The model under review builds one solid part; all positions refer to its coordinate system, in mm. Face numbers are marked on the shaded views. A direction names the side the tool comes from. Coordinates: 2 decimals unless noted, no trailing zeros. Loops run counter-clockwise (first coordinate to the right, second up) from the corner with the lowest first, then second, coordinate; pieces in that order, holes last. Notation, with made-up numbers: (-20, 54) - (8, 54) arc R27 cw to (8, 76) - close; hole circle Ø2 at (42.5, 68). An arc over 180 degrees is marked (long way). Use a Markdown table: item, result. Add a question column.
1) To check wall thickness, follow L1, parallel to X at y = 4, z = 14; L2, parallel to Z at x = 12, y = 7.5; L3, parallel to X at y = 80, z = 5.5. State the ranges of each line that lie inside material, in increasing order. Write a range as [from, to].
2) Add section A-A, the plane z = 14. Give the boundary of the cut face in (x, y), and give its area (3 significant figures).
3) Add section C-C, the plane x = 2.75. Give the boundary of the cut face in (y, z).
4) For the marked faces 1, 2 and 3, list the 3-axis set-ups (+Z, -Z, +X, -X, +Y, -Y) from which the entire face can be reached by the end or side of a thin tool; tool diameter is ignored.
5) Add section B-B, the plane x = 12. Give the boundary of the cut face in (y, z), and give its area (3 significant figures).
6) Clearance check with flat-ended pins moving along their axes: pin 1 (6 mm diameter, centred on y = 53.5, z = 7, fed in from +X); pin 2 (10 mm diameter, centred on y = 52.5, z = -0.5, fed in from -X); pin 3 (4 mm diameter, centred on x = 3.5, y = 72.5, fed in from +Z). State where each tip first meets the part, or that it passes through.
7) Add section D-D, the plane y = 41. Give the boundary of the cut face in (x, z), and give its area (3 significant figures).
```python
from build123d import *

# Parameters (mm, degrees)
BOSS_EXTRUDE2_DEPTH = 150
SKETCH3_W           = 29.65685425
SKETCH3_H           = 33.65685425
SKETCH3_R           = 2
BOSS_EXTRUDE3_DEPTH = 10


with BuildPart() as part:
    # Sketch1 → Boss-Extrude2 (new body)
    with BuildSketch(Plane(origin=(0, 0, 0), x_dir=(1, 0, 0), z_dir=(0, 1, 0))):
        Polygon((-10, 12.5), (-10, -12.5), (10, -12.5), (10, -5), (8, -5), (8, -8.6), (0, -8.6), (-6.2, -6), (-6.2, 0), (-6.2, 6), (0, 8.6), (8, 8.6), (8, 5), (10, 5), (10, 12.5), align=None)
    extrude(amount=BOSS_EXTRUDE2_DEPTH)

    # Sketch3 → Boss-Extrude3 (add)
    with BuildSketch(Plane(origin=(0, 0, 0), x_dir=(1, 0, 0), z_dir=(0, 1, 0))):
        Rectangle(SKETCH3_W, SKETCH3_H)
        with Locations(Location((-12, 14, 0), (0, 0, 270))):
            Circle(SKETCH3_R, mode=Mode.SUBTRACT)
        with Locations(Location((-12, -14, 0), (0, 0, 270))):
            Circle(SKETCH3_R, mode=Mode.SUBTRACT)
        with Locations(Location((12, 14, 0), (0, 0, 90))):
            Circle(SKETCH3_R, mode=Mode.SUBTRACT)
        with Locations(Location((12, -14, 0), (0, 0, 90))):
            Circle(SKETCH3_R, mode=Mode.SUBTRACT)
    extrude(amount=BOSS_EXTRUDE3_DEPTH)


solid = part.part
```
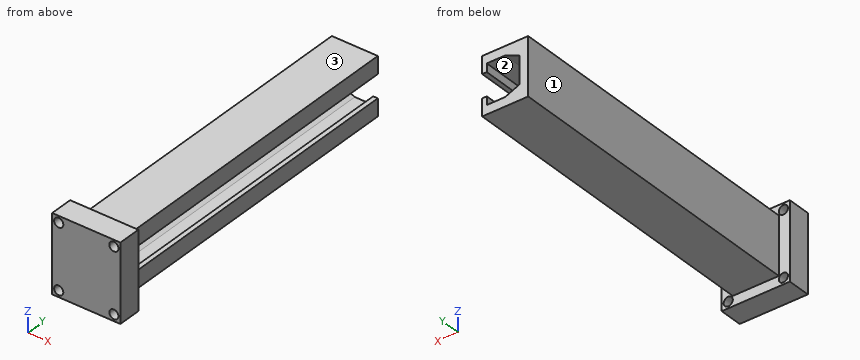
From the geometry:
| question | item | result |
|---|---|---|
| 1 | L1 | x = [-14.83, -14], [-10, 10], [14, 14.83] |
| 1 | L2 | z = [-16.83, -16], [-12, 12], [16, 16.83] |
| 1 | L3 | x = [-10, -6.2], [8, 10] |
| 2 | outline | (-14.83, 0) - (-14, 0) - (-14, 10) - (-14.83, 10) - close; (-10, 0) - (10, 0) - (10, 10) - (-10, 10) - close; (14, 0) - (14.83, 0) - (14.83, 10) - (14, 10) - close |
| 2 | area | 217 mm^2 |
| 3 | outline | (0, -16.83) - (10, -16.83) - (10, -12.5) - (150, -12.5) - (150, -8.6) - (10, -8.6) - (10, 8.6) - (150, 8.6) - (150, 12.5) - (10, 12.5) - (10, 16.83) - (0, 16.83) - close |
| 4 | face 1 | +Z, -Z, -X, +Y |
| 4 | face 2 | +Y |
| 4 | face 3 | +Z, +X, -X, +Y |
| 5 | outline | (0, -16.83) - (10, -16.83) - (10, -16) - (0, -16) - close; (0, -12) - (10, -12) - (10, 12) - (0, 12) - close; (0, 16) - (10, 16) - (10, 16.83) - (0, 16.83) - close |
| 5 | area | 257 mm^2 |
| 6 | pin 1 | stops at x = 10 |
| 6 | pin 2 | stops at x = -10 |
| 6 | pin 3 | stops at z = 12.5 |
| 7 | outline | (-10, -12.5) - (10, -12.5) - (10, -5) - (8, -5) - (8, -8.6) - (0, -8.6) - (-6.2, -6) - (-6.2, 6) - (0, 8.6) - (8, 8.6) - (8, 5) - (10, 5) - (10, 12.5) - (-10, 12.5) - close |
| 7 | area | 252 mm^2 |
